The model under review builds one solid part; all positions refer to its coordinate system, in mm. A direction names the side the tool comes from. Round coordinates to 2 decimals unless told otherwise and drop trailing zeros. Write each loop counter-clockwise with the first axis right and the second up, starting at its lowest first coordinate (ties: lowest second). Pieces come first, ordered by that corner, then holes. Notation, with made-up numbers: (70, 15) - (115, 15) arc R9 ccw to (115, 32) - close; hole circle Ø1 at (54.25, 85). An arc over 180 degrees is marked (long way). Use one line per item in the form item = value.
from build123d import *

# Parameters (mm, degrees)
SKETCH2_W           = 19
SKETCH2_H           = 15
BOSS_EXTRUDE1_DEPTH = 16
SKETCH3_W           = 18
SKETCH3_H           = 14
CUT_EXTRUDE1_DEPTH  = 1
CHAMFER1_SIZE       = 1
SKETCH4_R           = 0.5
BOSS_EXTRUDE3_DEPTH = 5
FILLET1_R           = 0.2


with BuildPart() as part:
    # Sketch2 → Boss-Extrude1 (new body)
    with BuildSketch(Plane(origin=(0, 0, 0), x_dir=(1, 0, 0), z_dir=(0, 1, 0))):
        Rectangle(SKETCH2_W, SKETCH2_H)
    extrude(amount=BOSS_EXTRUDE1_DEPTH)

    # Sketch3 → Cut-Extrude1 (cut)
    with BuildSketch(Plane(origin=(0, 16, 0), x_dir=(1, 0, 0), z_dir=(0, 1, 0))):
        Rectangle(SKETCH3_W, SKETCH3_H)
    extrude(amount=-CUT_EXTRUDE1_DEPTH, mode=Mode.SUBTRACT)

    # Chamfer1
    chamfer1_edges = [part.edges().sort_by_distance(p)[0] for p in [
        (0, 15, 7),
        (9, 15, 0),
        (0, 15, -7),
        (-9, 15, 0),
    ]]
    chamfer(chamfer1_edges, length=CHAMFER1_SIZE - 0.0001)  # a hair under: the kernel refuses the full size

    # Sketch4 → Boss-Extrude3 (add)
    with BuildSketch(Plane(origin=(0, 15, 0), x_dir=(1, 0, 0), z_dir=(0, 1, 0))):
        with Locations(Location((-8.1, 0, 0), (0, 0, 78.463040967))):
            Circle(SKETCH4_R)
        with Locations((-6.1, 6)):
            Circle(SKETCH4_R)
        with Locations((6.1, 6)):
            Circle(SKETCH4_R)
    boss_extrude3 = extrude(amount=BOSS_EXTRUDE3_DEPTH)

    # Mirror1: Boss-Extrude3 across plane
    add(boss_extrude3.mirror(Plane.XY))

    # Fillet1
    fillet1_edges = [part.edges().sort_by_distance(p)[0] for p in [
        (0, 0, 7.5),
        (-9.5, 0, 0),
        (0, 0, -7.5),
        (9.5, 0, 0),
        (9.5, 8, 7.5),
        (-9.5, 8, 7.5),
        (-9.5, 8, -7.5),
        (9.5, 8, -7.5),
    ]]
    fillet(fillet1_edges, radius=FILLET1_R)


solid = part.part
(1) To check wall thickness, follow L1, parallel to Z at x = -1, y = 15.5; L2, parallel to Y at x = -2.25, z = -4.75; L3, parallel to Z at x = -0.5, y = 15.25. State the ranges of each line that lie inside material, in increasing order.
Geometry results:
L1 = -7.5 to -6.5, 6.5 to 7.5
L2 = 0 to 15
L3 = -7.5 to -6.25, 6.25 to 7.5
(2) Add section D-D on y = 18.5. Write out the cut boundary in (x, z), then the cut area to 3 significant figures.
Geometry results:
outline = circle Ø1 at (-8.1, 0); circle Ø1 at (-6.1, -6); circle Ø1 at (-6.1, 6); circle Ø1 at (6.1, -6); circle Ø1 at (6.1, 6)
area = 3.93 mm2
(3) Add section A-A on y = 15.5. Write out the cut boundary in (x, z), then the cut area to 3 significant figures.
Geometry results:
outline = (-9.5, -7.3) arc R0.2 ccw to (-9.3, -7.5) - (9.3, -7.5) arc R0.2 ccw to (9.5, -7.3) - (9.5, 7.3) arc R0.2 ccw to (9.3, 7.5) - (-9.3, 7.5) arc R0.2 ccw to (-9.5, 7.3) - close; circle Ø1 at (-6.1, -6); circle Ø1 at (-6.1, 6); circle Ø1 at (6.1, -6); circle Ø1 at (6.1, 6); hole (-8.5, -6.5) - (8.5, -6.5) - (8.5, 6.5) - (-8.5, 6.5) - (-8.5, 0.3) arc R0.5 cw (long way) to (-8.5, -0.3) - close
area = 67.8 mm2
(4) Insertion check: P1, Ø1.5, axis at x = 6, z = 4, coming from the +Y side. The pin has a flat end and moves straight along its axis. Give the tip position at first contact, or say it passes through.
Geometry results:
P1 = 15
(5) The part is to be moulded in two halves that separate along Z. For faces 3 (the cylindrical face through (6.331, 17.465, 5.556)), 4 (the flat face through (-6, 20, 6)), 5 (the flat face through (0, 8, 7.5)), say which applies: +Z half, -Z half, draft (parallel to the pull), parting line (faces both ways), or undercut.
Geometry results:
face_3 = undercut
face_4 = draft
face_5 = +Z half
(6) Machinability: for faces 1 (the cylindrical face through (-5.869, 17.465, 5.556)), 2 (the flat face through (0, 8, -7.5)), which of the approach directions +Z, -Z, +X, -X, +Y, -Y give a long, thin tool a straight path to every point of the face, cutting with its end or side? Answer none if there is none.
Geometry results:
face_1 = +Y
face_2 = -Z, +X, -X, +Y, -Y
